Can you work these out from the model? Positions are in its coordinate system, mm. A direction names the side the tool comes from. Round coordinates to 2 decimals unless told otherwise and drop trailing zeros. Loops run counter-clockwise (first coordinate to the right, second up) from the corner with the lowest first, then second, coordinate; pieces in that order, holes last. Notation, with made-up numbers: (33.5, -19.5) -> (77.5, -19.5) arc R25 ccw to (77.5, -4.5) -> close; hole circle Ø4 at (-16, 19). An arc over 180 degrees is marked (long way). Answer as a JSON object with one key per item and string values.
```python
from build123d import *

# Parameters (mm, degrees)
SKETCH_1_R          = 3.05
SKETCH_1_R_2        = 1.05
EXTRUDE_1_DEPTH     = 3.5
SKETCH_2_W          = 16
SKETCH_2_H          = 36
EXTRUDE_2_DEPTH     = 3.5
EXTRUDE_4_DEPTH     = 3.5
EXTRUDE_5_DEPTH     = 8
CUT_EXTRUDE_1_REACH = 104.026
SKETCH_6_W          = 2.03
SKETCH_6_H          = 11.5
EXTRUDE_6_REACH     = 103.73
SKETCH_7_W          = 3
SKETCH_7_H          = 11.5
EXTRUDE_7_REACH     = 103.229
SKETCH_8_W          = 0.45
SKETCH_8_H          = 3.5
EXTRUDE_8_REACH     = 103.229
SKETCH_9_W          = 29
SKETCH_9_H          = 2
SKETCH_10_R         = 1.05
CUT_EXTRUDE_2_DEPTH = 31.75
CUT_EXTRUDE_3_DEPTH = 2
CUT_EXTRUDE_4_REACH = 88.626
SKETCH_13_W         = 11
SKETCH_13_H         = 10
SKETCH_14_W         = 13
SKETCH_14_H         = 28
CUT_EXTRUDE_5_DEPTH = 104.418337349
FILLET_1_R          = 1
CUT_EXTRUDE_6_DEPTH = 11.625
CUT_EXTRUDE_7_DEPTH = 10.125
CUT_EXTRUDE_8_DEPTH = 11.55


with BuildPart() as part:
    # Sketch 1 → Extrude 1 (new body)
    with BuildSketch(Plane(origin=(0, 0, 0), x_dir=(1, 0, 0), z_dir=(0, 1, 0))):
        with BuildLine():
            Line((0, 8), (-15, 8))
            Line((-15, 8), (-15, -8))
            Line((-15, -8), (0, -8))
            ThreePointArc((0, -8), (8, 0), (0, 8))
        make_face()
        with Locations(Location((0, 0, 0), (0, 0, 270))):
            Circle(SKETCH_1_R, mode=Mode.SUBTRACT)
        with Locations(Location((-4.242640687, 4.242640687, 0), (0, 0, 270))):
            Circle(SKETCH_1_R_2, mode=Mode.SUBTRACT)
        with Locations(Location((-4.242640687, -4.242640687, 0), (0, 0, 270))):
            Circle(SKETCH_1_R_2, mode=Mode.SUBTRACT)
        with Locations(Location((4.242640687, -4.242640687, 0), (0, 0, 90))):
            Circle(SKETCH_1_R_2, mode=Mode.SUBTRACT)
        with Locations(Location((4.242640687, 4.242640687, 0), (0, 0, 90))):
            Circle(SKETCH_1_R_2, mode=Mode.SUBTRACT)
    extrude(amount=EXTRUDE_1_DEPTH)


with BuildPart() as body_2:
    # Mirror 4: mirrored copy
    add(part.part.mirror(Plane.ZX.offset(18)))


with BuildPart() as part_1:
    add(part.part)

    add(body_2.part)  # Extrude 2 merges body 2
    # Sketch 2 → Extrude 2 (add)
    with BuildSketch(Plane.ZY.offset(15)):
        with Locations((0, 18)):
            Rectangle(SKETCH_2_W, SKETCH_2_H)
    extrude(amount=EXTRUDE_2_DEPTH)

    # Sketch 4 → Extrude 4 (add)
    with BuildSketch(Plane.XZ.offset(-32.5)):
        with BuildLine():
            Line((0, 8), (10.05, 8))
            Line((10.05, 8), (10.05, -8))
            Line((10.05, -8), (0, -8))
            ThreePointArc((0, -8), (8, 0), (0, 8))
        make_face()
    extrude(amount=-EXTRUDE_4_DEPTH)

    # Sketch 5 → Extrude 5 (add)
    with BuildSketch(Plane.XY.offset(8)):
        Polygon((10.05, 32.5), (-18.5, 32.5), (-18.95, 32.5), (-18.95, 96.5), (-18.5, 96.5), (10.05, 96.5), align=None)
    extrude_5 = extrude(amount=EXTRUDE_5_DEPTH)

    # Mirror 5: Extrude 5 across plane
    add(extrude_5.mirror(Plane.XY))

    # Sketch 6 → Cut-Extrude 1 (cut, up to next)
    with BuildSketch(Plane(origin=(10.05, 0, 0), x_dir=(0, 0, -1), z_dir=(1, 0, 0)), mode=Mode.PRIVATE) as cut_extrude_1_sk1:
        with Locations((-9.015, 90.75)):
            Rectangle(SKETCH_6_W, SKETCH_6_H)
    cut_extrude_1_tool1 = extrude(cut_extrude_1_sk1.sketch, amount=-CUT_EXTRUDE_1_REACH, mode=Mode.PRIVATE) & part_1.part
    # Sketch 6 → Cut-Extrude 1 (cut, up to next)
    with BuildSketch(Plane(origin=(10.05, 0, 0), x_dir=(0, 0, -1), z_dir=(1, 0, 0)), mode=Mode.PRIVATE) as cut_extrude_1_sk2:
        with Locations((9.015, 90.75)):
            Rectangle(SKETCH_6_W, SKETCH_6_H)
    cut_extrude_1_tool2 = extrude(cut_extrude_1_sk2.sketch, amount=-CUT_EXTRUDE_1_REACH, mode=Mode.PRIVATE) & part_1.part
    add(cut_extrude_1_tool1.solids().sort_by_distance((10.05, 90.75, 9.015))[0], mode=Mode.SUBTRACT)
    add(cut_extrude_1_tool2.solids().sort_by_distance((10.05, 90.75, -9.015))[0], mode=Mode.SUBTRACT)

    # Sketch 7 → Extrude 6 (add, up to next)
    with BuildSketch(Plane(origin=(0, 0, 10.03), x_dir=(-1, 0, 0), z_dir=(0, 0, -1)), mode=Mode.PRIVATE) as extrude_6_sk1:
        with Locations((17.45, 90.75)):
            Rectangle(SKETCH_7_W, SKETCH_7_H)
    extrude_6_tool1 = extrude(extrude_6_sk1.sketch, amount=EXTRUDE_6_REACH, mode=Mode.PRIVATE) - part_1.part
    # Sketch 7 → Extrude 6 (add, up to next)
    with BuildSketch(Plane(origin=(0, 0, 10.03), x_dir=(-1, 0, 0), z_dir=(0, 0, -1)), mode=Mode.PRIVATE) as extrude_6_sk2:
        with Locations((-8.55, 90.75)):
            Rectangle(SKETCH_7_W, SKETCH_7_H)
    extrude_6_tool2 = extrude(extrude_6_sk2.sketch, amount=EXTRUDE_6_REACH, mode=Mode.PRIVATE) - part_1.part
    add(extrude_6_tool1.solids().sort_by_distance((-17.45, 90.75, 10.03))[0])
    add(extrude_6_tool2.solids().sort_by_distance((8.55, 90.75, 10.03))[0])

    # Sketch 8 → Extrude 7 (add, up to next)
    with BuildSketch(Plane.XY.offset(-8), mode=Mode.PRIVATE) as extrude_7_sk1:
        with Locations((-18.725, 34.25)):
            Rectangle(SKETCH_8_W, SKETCH_8_H)
    extrude_7_tool1 = extrude(extrude_7_sk1.sketch, amount=EXTRUDE_7_REACH, mode=Mode.PRIVATE) - part_1.part
    add(extrude_7_tool1.solids().sort_by_distance((-18.725, 34.25, -8))[0])

    # Sketch 9 → Extrude 8 (add, up to next)
    with BuildSketch(Plane.XY.offset(-8), mode=Mode.PRIVATE) as extrude_8_sk1:
        with Locations((-4.45, 84)):
            Rectangle(SKETCH_9_W, SKETCH_9_H)
    extrude_8_tool1 = extrude(extrude_8_sk1.sketch, amount=EXTRUDE_8_REACH, mode=Mode.PRIVATE) - part_1.part
    add(extrude_8_tool1.solids().sort_by_distance((-4.45, 84, -8))[0])

    # Sketch 10 → Cut-Extrude 2 (cut, symmetric)
    with BuildSketch(Plane(origin=(-15.95, 0, 0), x_dir=(0, 0, -1), z_dir=(1, 0, 0))):
        with Locations(Location((-8, 87, 0), (0, 0, 180))):
            Circle(SKETCH_10_R)
        with Locations(Location((8, 87, 0), (0, 0, 180))):
            Circle(SKETCH_10_R)
    extrude(amount=CUT_EXTRUDE_2_DEPTH, both=True, mode=Mode.SUBTRACT)

    # Sketch 12 → Cut-Extrude 3 (cut)
    with BuildSketch(Plane(origin=(0, 3.5, 0), x_dir=(1, 0, 0), z_dir=(0, 1, 0))):
        with BuildLine():
            Line((0, 3.05), (11.782657366, 3.05))
            Line((11.782657366, 3.05), (11.782657366, -3.05))
            Line((11.782657366, -3.05), (0, -3.05))
            ThreePointArc((0, -3.05), (3.05, 0), (0, 3.05))
        make_face()
    extrude(amount=-CUT_EXTRUDE_3_DEPTH, mode=Mode.SUBTRACT)

    # Sketch 13 → Cut-Extrude 4 (cut, up to next)
    with BuildSketch(Plane.XZ.offset(-83), mode=Mode.PRIVATE) as cut_extrude_4_sk1:
        with Locations((-5.45, 0)):
            Rectangle(SKETCH_13_W, SKETCH_13_H)
    cut_extrude_4_tool1 = extrude(cut_extrude_4_sk1.sketch, amount=-CUT_EXTRUDE_4_REACH, mode=Mode.PRIVATE) & part_1.part
    add(cut_extrude_4_tool1.solids().sort_by_distance((-5.45, 83, 0))[0], mode=Mode.SUBTRACT)

    # Sketch 14 → Cut-Extrude 5 (cut, through all)
    with BuildSketch(Plane(origin=(0, 0, -16), x_dir=(-1, 0, 0), z_dir=(0, 0, -1))):
        with Locations((4.45, 62.5)):
            Rectangle(SKETCH_14_W, SKETCH_14_H)
    extrude(amount=-CUT_EXTRUDE_5_DEPTH, mode=Mode.SUBTRACT)

    # Fillet 1
    fillet_1_edges = [part_1.edges().sort_by_distance(p)[0] for p in [
        (-4.45, 96.5, -16),
        (10.05, 64.5, -16),
        (-4.45, 32.5, -16),
        (-18.95, 64.5, -16),
        (-4.45, 96.5, 10.03),
        (-4.45, 96.5, -10.03),
        (-15.95, 96.5, 0),
        (7.05, 96.5, 0),
        (-18.95, 36, 0),
        (-18.95, 59.5, 8),
        (-18.95, 59.5, -8),
        (-18.95, 83, 0),
        (10.05, 83, 0),
        (2.05, 62.5, 8),
        (2.05, 62.5, -8),
        (2.05, 62.5, 16),
        (-4.45, 76.5, 8),
        (-4.45, 76.5, -8),
        (-4.45, 76.5, 16),
        (-10.95, 62.5, 8),
        (-10.95, 62.5, -8),
        (-10.95, 62.5, 16),
        (-4.45, 48.5, 8),
        (-4.45, 48.5, -8),
        (-4.45, 48.5, 16),
        (-10.95, 62.5, -16),
        (-4.45, 76.5, -16),
        (10.05, 36, 0),
        (-18.95, 96.5, 0),
        (10.05, 59.5, 8),
        (10.05, 96.5, 0),
        (-4.45, 96.5, 16),
        (-18.95, 64.5, 16),
        (-4.45, 32.5, 16),
        (10.05, 64.5, 16),
        (10.05, 59.5, -8),
    ]]
    fillet(fillet_1_edges, radius=FILLET_1_R)

    # Sketch 16 → Cut-Extrude 6 (cut, symmetric)
    with BuildSketch(Plane.ZY.offset(4.45)):
        Polygon((-10.03, 95.5), (-10.03, 98.360674074), (10.03, 98.360674074), (10.03, 95.5), (10.03, 85), (-10.03, 85), align=None)
    extrude(amount=CUT_EXTRUDE_6_DEPTH, both=True, mode=Mode.SUBTRACT)

    # Sketch 17 → Cut-Extrude 7 (cut, symmetric)
    with BuildSketch(Plane.XY):
        Polygon((-16.075, 95.984122918), (-15.913726203, 99.204392549), (7.175, 98.048089827), (7.175, 95.984122918), (7.175, 85), (-16.075, 85), align=None)
    extrude(amount=CUT_EXTRUDE_7_DEPTH, both=True, mode=Mode.SUBTRACT)

    # Sketch 19 → Cut-Extrude 8 (cut, symmetric)
    with BuildSketch(Plane(origin=(-4.45, 0, 0), x_dir=(0, 0, -1), z_dir=(1, 0, 0))):
        Polygon((-10.125, 95.984122918), (-10.125, 99.965715237), (10.09, 99.965715237), (10.125, 95.984122918), (10.125, 85), (-10.125, 85), align=None)
    extrude(amount=CUT_EXTRUDE_8_DEPTH, both=True, mode=Mode.SUBTRACT)


solid = part_1.part
```
Q1. I want a section at C-C, the plane z = -13. Write out the boundary of the cut face in (x, y).
Determined:
{"outline": "(-18.95, 32.5) -> (10.05, 32.5) -> (10.05, 95.5) arc R1 ccw to (9.05, 96.5) -> (-17.95, 96.5) arc R1 ccw to (-18.95, 95.5) -> close; hole (-10.95, 48.5) -> (2.05, 48.5) -> (2.05, 76.5) -> (-10.95, 76.5) -> close"}
Q2. I want a section at B-B, the plane y = 87. Write out the boundary of the cut face in (x, z) (3 decimals).
Determined:
{"outline": "(-18.95, -15) arc R1 ccw to (-17.95, -16) -> (9.05, -16) arc R1 ccw to (10.05, -15) -> (10.05, -9.05) -> (7.175, -9.05) -> (7.175, -10.125) -> (-16.075, -10.125) -> (-16.075, -9.05) -> (-18.95, -9.05) -> close; (-18.95, -6.95) -> (-16.075, -6.95) -> (-16.075, 6.95) -> (-18.95, 6.95) -> close; (-18.95, 9.05) -> (-16.075, 9.05) -> (-16.075, 10.125) -> (7.175, 10.125) -> (7.175, 9.05) -> (10.05, 9.05) -> (10.05, 15) arc R1 ccw to (9.05, 16) -> (-17.95, 16) arc R1 ccw to (-18.95, 15) -> close; (7.175, -6.95) -> (10.05, -6.95) -> (10.05, 6.95) -> (7.175, 6.95) -> close"}
Q3. If I drill on L1, parallel to Y at x = -11.75, z = 3; L2, parallel to Z at x = 8.5, y = 87; L3, parallel to Y at x = -0.5, z = -4, over which ranges is the centre line in solid material (lowest first)? Write a range as [from, to].
Determined:
{"L1": "[0, 3.5], [32.5, 36], [83, 85]", "L2": "[-16, -9.05], [-6.95, 6.95], [9.05, 16]", "L3": "[0, 3.5], [32.5, 36]"}
Q4. I want a section at D-D, the plane y = 71. Give the number of separate pieces and of enclosed holes in the cut face, then the cut area to 3 significant figures.
Determined:
{"separate pieces": "4", "enclosed holes": "0", "area": "253 mm²"}
Q5. I'm going to push flat-ended pins straight in: pin 1 (10 mm diameter, centred on x = -1.5, z = 2, fed in from +Y); pin 2 (1.7 mm diameter, centred on y = 87, z = 8, fed in from -X); pin 3 (1.8 mm diameter, centred on x = -6.5, z = -13, fed in from -Y); pin 4 (1 mm diameter, centred on x = 5, y = 2.5, fed in from +Z). Where does each tip first touch, or does it pass through?
Determined:
{"pin 1": "y = 85", "pin 2": "through", "pin 3": "y = 32.5", "pin 4": "z = 6.61"}
Q6. On a 3-axis mill with a long thin cutter (end or side, diameter ignored), from which of +Z, -Z, +X, -X, +Y, -Y can I reach the whole of each face in a straight line? I mean faces 5 (the flat face through (4, 3, -3.05)), 6 (the flat face through (-15.5, 11.4, 8)), 7 (the flat face through (0.05, 84, 0)), 8 (the flat face through (-18.5, 16, 0)), 9 (the flat face through (-15.4, 11.4, -8)). Say none if no direction works.
Determined:
{"face 5": "+X", "face 6": "+Z, +X, -X, -Y", "face 7": "+Y", "face 8": "+Z, -Z, -X, -Y", "face 9": "-Z, +X, -X, -Y"}
Q7. We'd pull the mould along Z, two halves only. Please class faces 1 (the cylindrical face through (8.59, 85.96, 7.86)), 2 (the flat face through (5, 65, 16)), 3 (the cylindrical face through (-3.927, 1.726, 5.244)), 4 (the flat face through (-5, 48.5, -13)): pulls with the +Z half, pulls with the -Z half, needs draft (parallel to the pull), parting line crosses it, or undercut.
Determined:
{"face 1": "undercut", "face 2": "pulls with the +Z half", "face 3": "undercut", "face 4": "needs draft"}
Q8. I want a section at A-A, the plane x = -13.25. Write out the boundary of the cut face in (y, z) (3 decimals), then the cut area to 3 significant figures.
Determined:
{"outline": "(0, -8) -> (3.5, -8) -> (3.5, 8) -> (0, 8) -> close; (32.5, -15) arc R1 ccw to (33.5, -16) -> (95.5, -16) arc R1 ccw to (96.5, -15) -> (96.5, -11.03) arc R1 ccw to (95.925, -10.125) -> (85, -10.125) -> (85, 10.125) -> (95.925, 10.125) arc R1 ccw to (96.5, 11.03) -> (96.5, 15) arc R1 ccw to (95.5, 16) -> (33.5, 16) arc R1 ccw to (32.5, 15) -> close; hole (36, -8) -> (83, -8) -> (83, 8) -> (36, 8) -> close", "area": "1,120 mm²"}
